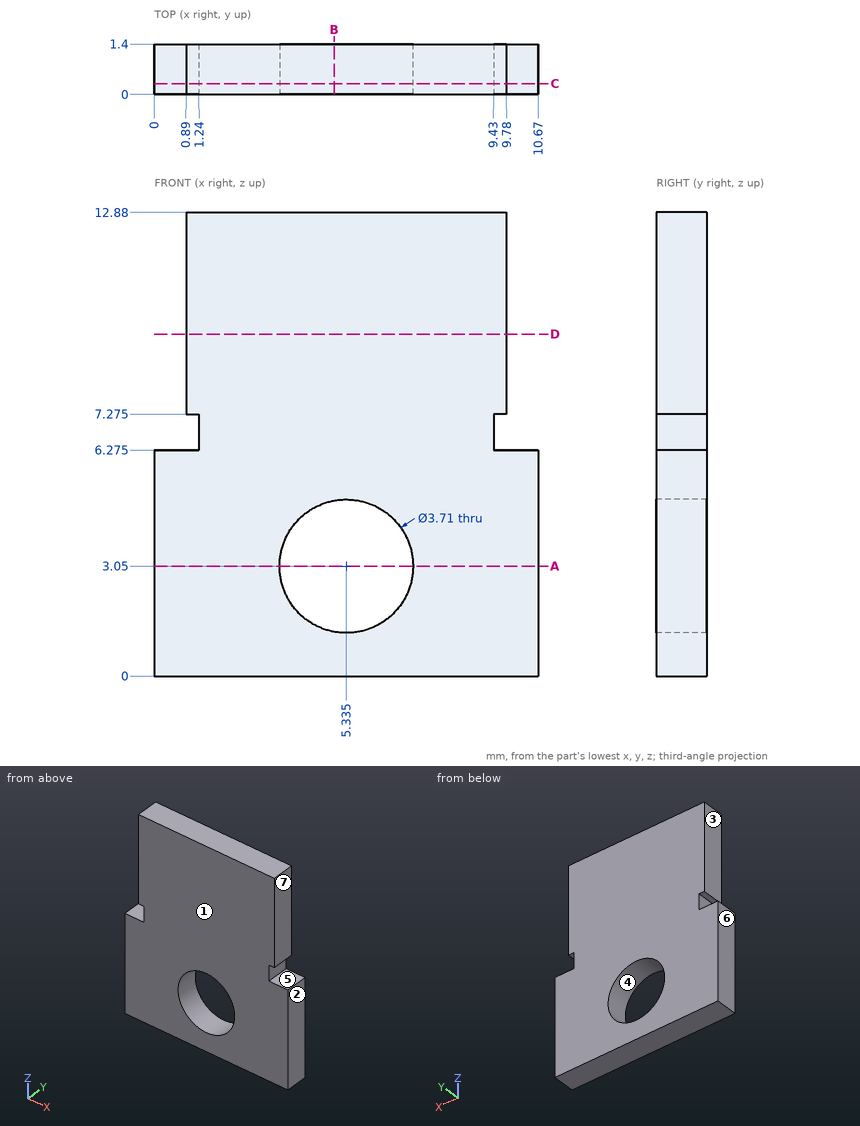
For this review, use the dimensioned drawing (mm, ordinates from the lowest corner) and the shaded views. A direction names the side the tool comes from. Round coordinates to 2 decimals unless told otherwise and drop trailing zeros. Order: outer loops, then holes, each group sorted by start corner. A loop starts at its lowest first (then second) coordinate and runs counter-clockwise, first axis right, second up.
1) Consider section A-A (z = 3.05). State the section outline as (x, y) points.
The answers:
outline: (0, 0) - (3.48, 0) - (3.48, 1.4) - (0, 1.4) - close; (7.19, 0) - (10.67, 0) - (10.67, 1.4) - (7.19, 1.4) - close
2) Consider section D-D (z = 9.5). State the section outline as (x, y) points.
The answers:
outline: (0.89, 0) - (9.78, 0) - (9.78, 1.4) - (0.89, 1.4) - close
3) For L1, parallel to Z at x = 1, y = 0.8 (3 decimals); L2, parallel to X at y = 0.95, z = 6.75; L3, parallel to Z at x = 4, y = 1.2, list the stretches that pass through material, from the lowest coordinate up.
The answers:
L1: z = 0 to 6.275, 7.275 to 12.88
L2: x = 1.24 to 9.43
L3: z = 0 to 1.76, 4.34 to 12.88
4) Draft analysis for pull direction X (two halves, no side actions). For the marked faces 1, 2, 3 and 4, state which applies: released by +X, released by -X, zero draft, split by the parting line, or undercut.
The answers:
face 1: zero draft
face 2: released by +X
face 3: released by -X
face 4: undercut
5) Clearance check with flat-ended pins moving along their axes: pin 1 Ø3.5 at (x, z) = (5.335, 3.05) entering from +Y; pin 2 Ø0.7 at (y, z) = (0.5, 10) entering from +X. State where each tip first meets the part, or that it passes through.
The answers:
pin 1: passes through
pin 2: stops at x = 9.78
6) Consider section B-B (x = 5). State the section outline as (y, z) points.
The answers:
outline: (0, 0) - (1.4, 0) - (1.4, 1.23) - (0, 1.23) - close; (0, 4.87) - (1.4, 4.87) - (1.4, 12.88) - (0, 12.88) - close
7) Machinability: for the marked faces 5, 6 and 7, which of the approach directions +Z, -Z, +X, -X, +Y, -Y give a long, thin tool a straight path to every point of the face, cutting with its end or side? Answer none if there is none.
The answers:
face 5: +X, +Y, -Y
face 6: +Z, -Z, -X, +Y, -Y
face 7: +Z, +X, +Y, -Y
8) Consider section C-C (y = 0.3). State the section outline as (x, z) points (3 decimals), plus the area to 3 significant figures.
The answers:
outline: (0, 0) - (10.67, 0) - (10.67, 6.275) - (9.43, 6.275) - (9.43, 7.275) - (9.78, 7.275) - (9.78, 12.88) - (0.89, 12.88) - (0.89, 7.275) - (1.24, 7.275) - (1.24, 6.275) - (0, 6.275) - close; hole circle Ø3.71 at (5.335, 3.05)
area: 114 mm2
